Source: CAD feature listing. Evaluate the final solid. Frame: model axes, mm. A direction names the side the tool comes from. Coordinates: 2 decimals unless noted, no trailing zeros. Order: outer loops, then holes, each group sorted by start corner. A loop starts at its lowest first (then second) coordinate and runs counter-clockwise, first axis right, second up.
```python
from build123d import *

# Parameters (mm, degrees)
SKETCH_R     = 16.75
PAD_DEPTH    = 3.6
SKETCH003_R  = 9.5
PAD002_DEPTH = 5.5
SKETCH001_R  = 4.5
PAD001_DEPTH = 3
SKETCH002_R  = 2.75
POCKET_DEPTH = 12.101


with BuildPart() as part:
    # Sketch → Pad (new body)
    with BuildSketch(Plane.XY):
        Circle(SKETCH_R)
    extrude(amount=PAD_DEPTH)

    # Sketch003 (on Face2 of Pocket) → Pad002 (join)
    with BuildSketch(Plane(origin=(0, 0, 0), x_dir=(1, 0, 0), z_dir=(0, 0, -1))):
        Circle(SKETCH003_R)
    extrude(amount=PAD002_DEPTH)

    # Sketch001 (on Face3 of Pad) → Pad001 (join)
    with BuildSketch(Plane.XY.offset(3.6)):
        Circle(SKETCH001_R)
    extrude(amount=PAD001_DEPTH)

    # Sketch002 (on Face5 of Pad001) → Pocket (cut, through all)
    with BuildSketch(Plane.XY.offset(6.6)):
        Circle(SKETCH002_R)
    extrude(amount=-POCKET_DEPTH, mode=Mode.SUBTRACT)


solid = part.part
```
Q1. Set-up query: faces 4 (the flat face through (7, -7, 0)), 5 (the flat face through (2, -2.2, -5.5)), 6 (the cylindrical face through (-0.59, 4.46, 5.08)). Return all of +Z, -Z, +X, -X, +Y, -Y with unobstructed straight access to the full face (end or side cutting, diameter ignored); none if empty.
Solutions:
face 4: -Z
face 5: -Z, +X, -X, +Y, -Y
face 6: +Z
Q2. Section query C-C on z = 0.5. Output: boundary loops of the cut face in (x, y).
Solutions:
outline: circle Ø33.5 at (0, 0); hole circle Ø5.5 at (0, 0)
Q3. Pin query (flat end, axial travel): P1, Ø4, axis at y = 12.5, z = -0.5, coming from the +X side; P2, Ø10, axis at x = -10.5, y = 13, coming from the -Z side; P3, Ø5, axis at y = 3, z = -1.5, coming from the +X side. Return the tip coordinate at first contact, or that it passes through.
Solutions:
P1: stops at x = 13
P2: stops at z = 0
P3: stops at x = 16.72
Q4. Section query D-D on x = -8.5. Output: boundary loops of the cut face in (y, z), plus the area to 3 significant figures.
Solutions:
outline: (-14.43, 0) - (-4.24, 0) - (-4.24, -5.5) - (4.24, -5.5) - (4.24, 0) - (14.43, 0) - (14.43, 3.6) - (-14.43, 3.6) - close
area: 151 mm2
Q5. Material intervals for line 1 along Y through (x, z) = (0, 0.75); line 2 along Y through (x, z) = (0, -3); line 3 along Z through (x, y) = (4, -12), sorted ascending.
Solutions:
line 1: y = -16.75 to -2.75, 2.75 to 16.75
line 2: y = -9.5 to -2.75, 2.75 to 9.5
line 3: z = 0 to 3.6
Q6. Section query A-A on x = 0. Output: boundary loops of the cut face in (y, z).
Solutions:
outline: (-16.75, 0) - (-9.5, 0) - (-9.5, -5.5) - (-2.75, -5.5) - (-2.75, 6.6) - (-4.5, 6.6) - (-4.5, 3.6) - (-16.75, 3.6) - close; (2.75, -5.5) - (9.5, -5.5) - (9.5, 0) - (16.75, 0) - (16.75, 3.6) - (4.5, 3.6) - (4.5, 6.6) - (2.75, 6.6) - close
Q7. Pull-direction query (X, two-part tool) for faces 1 (the flat face through (0, -3, 6.6)), 2 (the cylindrical face through (4.38, 8.43, -2.71)), 3 (the cylindrical face through (-0.596, -2.685, 0.635)); classes: pulls with the +X half, pulls with the -X half, needs draft (parallel to the pull), parting line crosses it, or undercut.
Solutions:
face 1: needs draft
face 2: parting line crosses it
face 3: undercut
